Check sheet for the drawn part. Datum: minimum x, y, z corner. Units: mm. A direction names the side the tool comes from. Coordinates: 2 decimals unless noted, no trailing zeros. Loops run counter-clockwise (first coordinate to the right, second up) from the corner with the lowest first, then second, coordinate; pieces in that order, holes last.
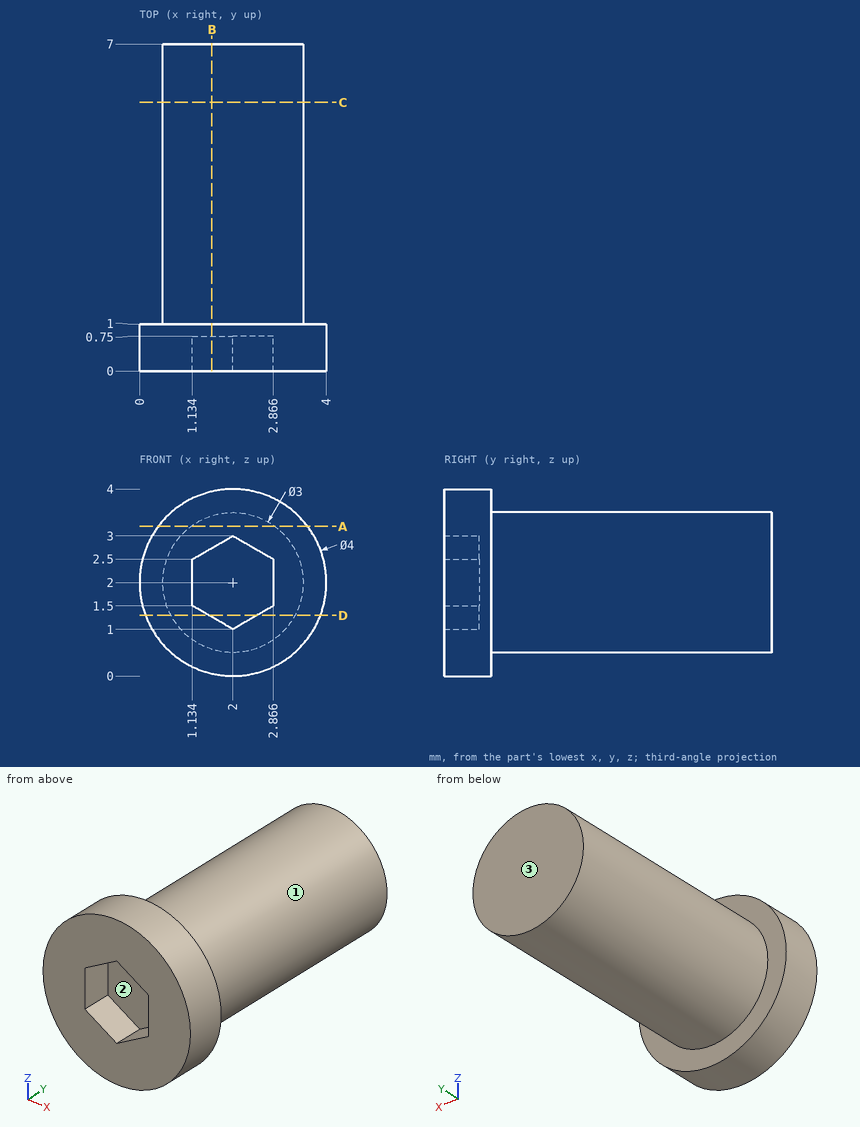
1) Set-up check for the marked faces 1, 2 and 3: record each of +Z, -Z, +X, -X, +Y, -Y from which the full face is reachable in a straight line by a thin tool's end or side.
Answer sheet:
face 1: +Y
face 2: -Y
face 3: +Z, -Z, +X, -X, +Y
2) Section check B-B on x = 1.55. Enter the section's corners in (y, z), plus the area to 3 significant figures.
Answer sheet:
outline: (0, 0.05) - (1, 0.05) - (1, 0.57) - (7, 0.57) - (7, 3.43) - (1, 3.43) - (1, 3.95) - (0, 3.95) - (0, 2.74) - (0.75, 2.74) - (0.75, 1.26) - (0, 1.26) - close
area: 20.0 mm2
3) Section check C-C on y = 5.75. Enter the section's corners in (x, z), plus the area to 3 significant figures.
Answer sheet:
outline: circle Ø3 at (2, 2)
area: 7.07 mm2
4) Section check D-D on z = 1.3. Enter the section's corners in (x, y).
Answer sheet:
outline: (0.13, 0) - (1.48, 0) - (1.48, 0.75) - (2.52, 0.75) - (2.52, 0) - (3.87, 0) - (3.87, 1) - (3.33, 1) - (3.33, 7) - (0.67, 7) - (0.67, 1) - (0.13, 1) - close
5) Scan lines: line 1 (Y direction, x = 1.6, z = 2.65); line 2 (X direction, y = 0.5, z = 1.6); line 3 (Y direction, x = 2.5, z = 3.55). Record each from-to range of solid material in increasing order.
Answer sheet:
line 1: y = 0.75 to 7
line 2: x = 0.04 to 1.13, 2.87 to 3.96
line 3: y = 0 to 1
6) Section check A-A on z = 3.2. Enter the section's corners in (x, y), plus the area to 3 significant figures.
Answer sheet:
outline: (0.4, 0) - (3.6, 0) - (3.6, 1) - (2.9, 1) - (2.9, 7) - (1.1, 7) - (1.1, 1) - (0.4, 1) - close
area: 14.0 mm2
7) Depth check by flat-ended pin: pin 1 (1 mm diameter, centred on x = 1.5, y = 4.5, fed in from -Z). Enter the tip coordinate at first touch or a pass-through.
Answer sheet:
pin 1: stops at z = 0.5
